Work out the finished part from the listing and answer in its coordinate system (mm). Give positions to 0.01 mm unless a question says otherwise; leave off trailing zeros. Order: outer loops, then holes, each group sorted by start corner. A loop starts at its lowest first (then second) coordinate and runs counter-clockwise, first axis right, second up.
```python
from build123d import *

# Parameters (mm, degrees)
BOSS_EXTRUDE1_DEPTH            = 1.6002
SKETCH3_W                      = 165.1
SKETCH3_H                      = 9.525
CUT_EXTRUDE1_DEPTH             = 295.167716856
FILLET1_R                      = 3.175
FUSE_ZIPTIE_MOUNTS_DEPTH       = 295.167716856
SKETCH5_R                      = 2.75
CONTACTOR_MOUNTING_HOLES_DEPTH = 295.167716856
SKETCH6_R                      = 1.8288
CUT_EXTRUDE2_DEPTH             = 295.167716856
SKETCH7_R                      = 2.7051
CUT_EXTRUDE3_DEPTH             = 295.167716856


with BuildPart() as part:
    # Sketch1 → Boss-Extrude1 (new body)
    with BuildSketch(Plane(origin=(0, 0, 0), x_dir=(1, 0, 0), z_dir=(0, 1, 0))):
        Polygon((0, 0), (247.65, 0), (247.65, 158.75), (50.8, 158.75), (50.8, 120.65), (0, 120.65), align=None)
    extrude(amount=BOSS_EXTRUDE1_DEPTH)

    # Sketch3 → Cut-Extrude1 (cut, through all)
    with BuildSketch(Plane(origin=(0, 1.6002, 0), x_dir=(1, 0, 0), z_dir=(0, 1, 0))):
        with Locations((165.1, 4.7625)):
            Rectangle(SKETCH3_W, SKETCH3_H)
    extrude(amount=-CUT_EXTRUDE1_DEPTH, mode=Mode.SUBTRACT)

    # Fillet1
    fillet1_edges = [part.edges().sort_by_distance(p)[0] for p in [
        (247.65, 0.8001, -158.75),
        (0, 0.8001, 0),
        (0, 0.8001, -120.65),
        (50.8, 0.8001, -120.65),
        (50.8, 0.8001, -158.75),
        (82.55, 0.8001, 0),
        (82.55, 0.8001, -9.525),
        (247.65, 0.8001, -9.525),
    ]]
    fillet(fillet1_edges, radius=FILLET1_R)

    # Sketch4 → Fuse Ziptie Mounts (cut, through all)
    with BuildSketch(Plane(origin=(0, 1.6002, 0), x_dir=(1, 0, 0), z_dir=(0, 1, 0))):
        with BuildLine():
            Line((165.653, 154.225), (168.193, 154.225))
            ThreePointArc((168.193, 154.225), (170.098, 152.32), (168.193, 150.415))
            Line((168.193, 150.415), (165.653, 150.415))
            ThreePointArc((165.653, 150.415), (163.748, 152.32), (165.653, 154.225))
        make_face()
        with BuildLine():
            Line((203.753, 154.225), (206.293, 154.225))
            ThreePointArc((206.293, 154.225), (208.198, 152.32), (206.293, 150.415))
            Line((206.293, 150.415), (203.753, 150.415))
            ThreePointArc((203.753, 150.415), (201.848, 152.32), (203.753, 154.225))
        make_face()
        with BuildLine():
            Line((203.753, 125.015), (206.293, 125.015))
            ThreePointArc((206.293, 125.015), (208.198, 123.11), (206.293, 121.205))
            Line((206.293, 121.205), (203.753, 121.205))
            ThreePointArc((203.753, 121.205), (201.848, 123.11), (203.753, 125.015))
        make_face()
        with BuildLine():
            Line((165.653, 125.015), (168.193, 125.015))
            ThreePointArc((168.193, 125.015), (170.098, 123.11), (168.193, 121.205))
            Line((168.193, 121.205), (165.653, 121.205))
            ThreePointArc((165.653, 121.205), (163.748, 123.11), (165.653, 125.015))
        make_face()
    extrude(amount=-FUSE_ZIPTIE_MOUNTS_DEPTH, mode=Mode.SUBTRACT)

    # Sketch5 → Contactor Mounting Holes (cut, through all)
    with BuildSketch(Plane(origin=(0, 1.6002, 0), x_dir=(1, 0, 0), z_dir=(0, 1, 0))):
        with Locations(Location((99.298, 103.9876, 0), (0, 0, 270))):
            Circle(SKETCH5_R)
        with Locations(Location((99.298, 35.7124, 0), (0, 0, 270))):
            Circle(SKETCH5_R)
        with Locations(Location((169.148, 103.9876, 0), (0, 0, 270))):
            Circle(SKETCH5_R)
        with Locations(Location((169.148, 35.7124, 0), (0, 0, 270))):
            Circle(SKETCH5_R)
    extrude(amount=-CONTACTOR_MOUNTING_HOLES_DEPTH, mode=Mode.SUBTRACT)

    # Sketch6 → Cut-Extrude2 (cut, through all)
    with BuildSketch(Plane(origin=(0, 1.6002, 0), x_dir=(1, 0, 0), z_dir=(0, 1, 0))):
        with Locations(Location((6.35, 114.3, 0), (0, 0, 270))):
            Circle(SKETCH6_R)
        with Locations(Location((76.2, 6.35, 0), (0, 0, 270))):
            Circle(SKETCH6_R)
        with Locations(Location((241.3, 15.875, 0), (0, 0, 270))):
            Circle(SKETCH6_R)
        with Locations(Location((241.3, 120.65, 0), (0, 0, 270))):
            Circle(SKETCH6_R)
        with Locations(Location((57.15, 133.35, 0), (0, 0, 270))):
            Circle(SKETCH6_R)
    extrude(amount=-CUT_EXTRUDE2_DEPTH, mode=Mode.SUBTRACT)

    # Sketch7 → Cut-Extrude3 (cut, through all)
    with BuildSketch(Plane(origin=(0, 1.6002, 0), x_dir=(1, 0, 0), z_dir=(0, 1, 0))):
        with Locations(Location((11.198, 102.95, 0), (0, 0, 270))):
            Circle(SKETCH7_R)
        with Locations(Location((56.198, 102.95, 0), (0, 0, 270))):
            Circle(SKETCH7_R)
        with Locations(Location((11.198, 12.95, 0), (0, 0, 270))):
            Circle(SKETCH7_R)
        with Locations(Location((56.198, 12.95, 0), (0, 0, 270))):
            Circle(SKETCH7_R)
    extrude(amount=-CUT_EXTRUDE3_DEPTH, mode=Mode.SUBTRACT)


solid = part.part
```
1. Given P1, Ø7, axis at x = 169.15, z = -103.99, coming from the +Y side; P2, Ø3.5, axis at x = 57.15, z = -133.35, coming from the +Y side; P3, Ø0.5, axis at x = 167.5, y = 1, coming from the +Z side (3 decimals); P4, Ø0.5, axis at x = 17, y = 1, coming from the -Z side, each flat-ended and moving along its own axis, determine where each tip first touches the part or whether it passes through.
Findings below:
P1: stops at y = 1.6
P2: passes through
P3: stops at z = -9.525
P4: stops at z = -120.65
2. Straight lines are drawn through the part: probe 1 along X at (y, z) = (0.65, -13); probe 2 along X at (y, z) = (0.85, -36); probe 3 along Z at (x, y) = (241.3, 0.4) (3 decimals). For each, find the intervals that lie inside material, in ascending order.
Findings below:
probe 1: x = 0 to 8.49, 13.9 to 53.49, 58.9 to 247.65
probe 2: x = 0 to 96.56, 102.03 to 166.41, 171.88 to 247.65
probe 3: z = -158.75 to -122.479, -118.821 to -17.704, -14.046 to -9.525
3. The part is cut by section B-B (y = 0.35). State how many separate pieces and enclosed holes the cut face has, then the cut area to 3 significant figures.
Findings below:
separate pieces: 1
enclosed holes: 17
area: 35,500 mm2
4. The mould has two halves that part along Z. Classify faces 1 (the face through (122, 1.6, -80)), 2 (the face through (101.617, 0.811, -102.509)): pulls with the +Z half, pulls with the -Z half, needs draft (parallel to the pull), parting line crosses it, or undercut.
Findings below:
face 1: needs draft
face 2: undercut
5. The part is cut by section A-A (z = -128). Write down the section's boundary in (x, y), then the cut area to 3 significant figures.
Findings below:
outline: (50.8, 0) - (247.65, 0) - (247.65, 1.6) - (50.8, 1.6) - close
area: 315 mm2
